Verification items for the finished model (mm, model axes). A direction names the side the tool comes from. Coordinates: 2 decimals unless noted, no trailing zeros. Write each loop counter-clockwise with the first axis right and the second up, starting at its lowest first coordinate (ties: lowest second). Pieces come first, ordered by that corner, then holes.
```python
from build123d import *

# Parameters (mm, degrees)
BOSS_EXTRU_1_DEPTH = 0.01
BOSS_EXTRU_2_DEPTH = 1.8
BOSS_EXTRU_3_DEPTH = 1.6
ESQUISSE4_R        = 2
ESQUISSE4_R_2      = 1
BOSS_EXTRU_4_DEPTH = 2.5


with BuildPart() as part:
    # Esquisse1 → Boss.-Extru.1 (new body)
    with BuildSketch(Plane.XY):
        with BuildLine():
            Line((-11.315, -13.985), (11.315, -13.985))
            ThreePointArc((11.315, -13.985), (14.850533906, -12.520533906), (16.315, -8.985))
            Line((16.315, -8.985), (16.315, 8.985))
            ThreePointArc((16.315, 8.985), (14.850533906, 12.520533906), (11.315, 13.985))
            Line((11.315, 13.985), (-11.315, 13.985))
            ThreePointArc((-11.315, 13.985), (-14.850533906, 12.520533906), (-16.315, 8.985))
            Line((-16.315, 8.985), (-16.315, -8.985))
            ThreePointArc((-16.315, -8.985), (-14.850533906, -12.520533906), (-11.315, -13.985))
        make_face()
    extrude(amount=-BOSS_EXTRU_1_DEPTH)

    # Esquisse2 → Boss.-Extru.2 (add)
    with BuildSketch(Plane(origin=(0, 0, -0.01), x_dir=(-1, 0, 0), z_dir=(0, 0, -1))):
        with BuildLine():
            Line((-15.015, -15.035), (12.415, -15.035))
            ThreePointArc((12.415, -15.035), (15.950533906, -13.570533906), (17.415, -10.035))
            Line((17.415, -10.035), (17.415, 10.035))
            ThreePointArc((17.415, 10.035), (15.950533906, 13.570533906), (12.415, 15.035))
            Line((12.415, 15.035), (-15.015, 15.035))
            ThreePointArc((-15.015, 15.035), (-18.550533906, 13.570533906), (-20.015, 10.035))
            Line((-20.015, 10.035), (-20.015, -10.035))
            ThreePointArc((-20.015, -10.035), (-18.550533906, -13.570533906), (-15.015, -15.035))
        make_face()
    extrude(amount=BOSS_EXTRU_2_DEPTH)

    # Esquisse3 → Boss.-Extru.3 (add)
    with BuildSketch(Plane(origin=(0, 0, -1.81), x_dir=(-1, 0, 0), z_dir=(0, 0, -1))):
        with BuildLine():
            Line((-15.3, -15.75), (12.7, -15.75))
            ThreePointArc((12.7, -15.75), (16.589087297, -14.139087297), (18.2, -10.25))
            Line((18.2, -10.25), (18.2, 10.25))
            ThreePointArc((18.2, 10.25), (16.589087297, 14.139087297), (12.7, 15.75))
            Line((12.7, 15.75), (-15.3, 15.75))
            ThreePointArc((-15.3, 15.75), (-19.189087297, 14.139087297), (-20.8, 10.25))
            Line((-20.8, 10.25), (-20.8, -10.25))
            ThreePointArc((-20.8, -10.25), (-19.189087297, -14.139087297), (-15.3, -15.75))
        make_face()
    extrude(amount=BOSS_EXTRU_3_DEPTH)

    # Esquisse4 → Boss.-Extru.4 (add)
    # profile 1 of 4: a face of its own
    with BuildSketch(Plane(origin=(0, 0, -3.41), x_dir=(-1, 0, 0), z_dir=(0, 0, -1))):
        with Locations(Location((-17.2, -12.15, 0), (0, 0, 180))):
            Circle(ESQUISSE4_R)
        with Locations((-17.2, -12.15)):
            Circle(ESQUISSE4_R_2, mode=Mode.SUBTRACT)
    # profile 2 of 4: a face of its own
    with BuildSketch(Plane(origin=(0, 0, -3.41), x_dir=(-1, 0, 0), z_dir=(0, 0, -1))):
        with Locations(Location((14.6, -12.15, 0), (0, 0, 180))):
            Circle(ESQUISSE4_R)
        with Locations((14.6, -12.15)):
            Circle(ESQUISSE4_R_2, mode=Mode.SUBTRACT)
    # profile 3 of 4: a face of its own
    with BuildSketch(Plane(origin=(0, 0, -3.41), x_dir=(-1, 0, 0), z_dir=(0, 0, -1))):
        with Locations(Location((-17.2, 12.15, 0), (0, 0, 180))):
            Circle(ESQUISSE4_R)
        with Locations((-17.2, 12.15)):
            Circle(ESQUISSE4_R_2, mode=Mode.SUBTRACT)
    # profile 4 of 4: a face of its own
    with BuildSketch(Plane(origin=(0, 0, -3.41), x_dir=(-1, 0, 0), z_dir=(0, 0, -1))):
        with Locations(Location((14.6, 12.15, 0), (0, 0, 180))):
            Circle(ESQUISSE4_R)
        with Locations((14.6, 12.15)):
            Circle(ESQUISSE4_R_2, mode=Mode.SUBTRACT)
    extrude(amount=BOSS_EXTRU_4_DEPTH)


solid = part.part
```
1. Gauge pin test, flat ends, axial feed: P1, Ø0.9, axis at y = -1.5, z = -0.5, coming from the -X side (3 decimals); P2, Ø1, axis at x = 17, y = 11.5, coming from the -Z side; P3, Ø1, axis at y = 9, z = -4.5, coming from the +X side; P4, Ø4, axis at x = -5.5, y = -12, coming from the -Z side. Record the tip position at first contact, or that the pin passes through.
2. Tool access check on faces 4 (the flat face through (-15, -12, -3.41)), 5 (the flat face through (20.015, 0, -1)), 6 (the flat face through (1, -15.75, -3)), 7 (the cylindrical face through (18.51, 13.61, -0.9)), 8 (the flat face through (1, 15.035, -1)). Record the directions out of +Z, -Z, +X, -X, +Y, -Y that give a thin tool (end or side, any length) a straight path to the whole face; none if there is none.
3. Sectioned sample at B-B, the plane z = -2.9. Record the boundary of the cut face in (x, y).
4. Sectioned sample at A-A, the plane z = -5.15. Record the boundary of the cut face in (x, y).
5. Draft check along X on faces 1 (the flat face through (16, -12, -5.91)), 2 (the cylindrical face through (-15.99, 13.53, -0.9)), 3 (the cylindrical face through (16.94, 10.167, -4.642)). Enter one of: pulls with the +X half, pulls with the -X half, needs draft (parallel to the pull), parting line crosses it, or undercut.
6. Material ranges on L1, parallel to Y at x = -14.6, z = -4.2; L2, parallel to Z at x = 3, y = -11; L3, parallel to Y at x = 1.5, z = -0.55 (3 decimals), recorded low to high.
7. Sectioned sample at C-C, the plane x = -9. Record the boundary of the cut face in (y, z) (3 decimals).
Outcome:
1. P1: stops at x = -17.415
1. P2: stops at z = -5.91
1. P3: passes through
1. P4: stops at z = -3.41
2. face 4: -Z
2. face 5: +Z, +X, +Y, -Y
2. face 6: +Z, -Z, +X, -X, -Y
2. face 7: +Z, +X, +Y
2. face 8: +Z, +X, -X, +Y
3. outline: (-18.2, -10.25) arc R5.5 ccw to (-12.7, -15.75) - (15.3, -15.75) arc R5.5 ccw to (20.8, -10.25) - (20.8, 10.25) arc R5.5 ccw to (15.3, 15.75) - (-12.7, 15.75) arc R5.5 ccw to (-18.2, 10.25) - close
4. outline: circle Ø4 at (-14.6, -12.15); circle Ø4 at (-14.6, 12.15); circle Ø4 at (17.2, -12.15); circle Ø4 at (17.2, 12.15); hole circle Ø2 at (-14.6, -12.15); hole circle Ø2 at (-14.6, 12.15); hole circle Ø2 at (17.2, -12.15); hole circle Ø2 at (17.2, 12.15)
5. face 1: needs draft
5. face 2: pulls with the -X half
5. face 3: undercut
6. L1: y = -14.15 to -13.15, -11.15 to -10.15, 10.15 to 11.15, 13.15 to 14.15
6. L2: z = -3.41 to 0
6. L3: y = -15.035 to 15.035
7. outline: (-15.75, -3.41) - (15.75, -3.41) - (15.75, -1.81) - (15.035, -1.81) - (15.035, -0.01) - (13.985, -0.01) - (13.985, 0) - (-13.985, 0) - (-13.985, -0.01) - (-15.035, -0.01) - (-15.035, -1.81) - (-15.75, -1.81) - close
